For this review, take the finished solid that the model builds, in its own axes (mm). A direction names the side the tool comes from. Coordinates: 2 decimals unless noted, no trailing zeros. Write each loop counter-clockwise with the first axis right and the second up, starting at its lowest first coordinate (ties: lowest second). Pieces come first, ordered by that corner, then holes.
```python
from build123d import *

# Parameters (mm, degrees)
SKETCH_1_W          = 50
SKETCH_1_H          = 29.5
SKETCH_1_R          = 1.75
EXTRUDE_1_DEPTH     = 5
SKETCH_1_17_R       = 3.1
CUT_EXTRUDE_1_DEPTH = 2.6
EXTRUDE_START       = 5
SKETCH_1_18_W       = 50
SKETCH_1_18_H       = 4
SKETCH_1_18_W_2     = 15
EXTRUDE_2_DEPTH     = 49
SKETCH_2_R          = 1.5
CUT_EXTRUDE_2_DEPTH = 76.968743573
SKETCH_2_4_R        = 2.25
CUT_EXTRUDE_3_DEPTH = 2
SKETCH_4_R          = 1.5
CUT_EXTRUDE_4_DEPTH = 75.553671942
SKETCH_4_3_R        = 2.25
CUT_EXTRUDE_5_DEPTH = 2
SKETCH_5_W          = 35
SKETCH_5_H          = 4
EXTRUDE_4_DEPTH     = 32
SKETCH_6_R          = 1.5
CUT_EXTRUDE_6_DEPTH = 97.944571792
SKETCH_6_3_R        = 2.25
CUT_EXTRUDE_7_DEPTH = 2


with BuildPart() as part:
    # 草图1 → 凸台-拉伸1 (new body)
    with BuildSketch(Plane(origin=(0, 0, 0), x_dir=(1, 0, 0), z_dir=(0, 1, 0))):
        with Locations((25, -14.75)):
            Rectangle(SKETCH_1_W, SKETCH_1_H)
        with Locations(Location((23.4, -12, 0), (0, 0, 270))):
            Circle(SKETCH_1_R, mode=Mode.SUBTRACT)
        with Locations(Location((44.400952359, -19.4, 0), (0, 0, 270))):
            Circle(SKETCH_1_R, mode=Mode.SUBTRACT)
    extrude(amount=EXTRUDE_1_DEPTH)

    # 草图1<17> → 切除-拉伸1 (cut)
    with BuildSketch(Plane(origin=(0, 0, 0), x_dir=(1, 0, 0), z_dir=(0, 1, 0))):
        with Locations(Location((23.4, -12, 0), (0, 0, 270))):
            Circle(SKETCH_1_17_R)
        with Locations(Location((44.400952359, -19.4, 0), (0, 0, 270))):
            Circle(SKETCH_1_17_R)
    extrude(amount=CUT_EXTRUDE_1_DEPTH, mode=Mode.SUBTRACT)

    # 草图1<18> → 凸台-拉伸2 (add)
    with BuildSketch(Plane(origin=(0, 0, 0), x_dir=(1, 0, 0), z_dir=(0, 1, 0)).offset(EXTRUDE_START)):
        with Locations((25, 2)):
            Rectangle(SKETCH_1_18_W, SKETCH_1_18_H)
        with Locations((7.5, 2)):
            Rectangle(SKETCH_1_18_W_2, SKETCH_1_18_H)
    extrude(amount=-EXTRUDE_2_DEPTH)

    # 草图2 → 切除-拉伸2 (cut, through all)
    with BuildSketch(Plane(origin=(0, 5, 0), x_dir=(1, 0, 0), z_dir=(0, 1, 0))):
        with Locations(Location((5, -24.5, 0), (0, 0, 270))):
            Circle(SKETCH_2_R)
        with Locations(Location((5, -6, 0), (0, 0, 270))):
            Circle(SKETCH_2_R)
    extrude(amount=-CUT_EXTRUDE_2_DEPTH, mode=Mode.SUBTRACT)

    # 草图2<4> → 切除-拉伸3 (cut)
    with BuildSketch(Plane(origin=(0, 5, 0), x_dir=(1, 0, 0), z_dir=(0, 1, 0))):
        with Locations(Location((5, -24.5, 0), (0, 0, 270))):
            Circle(SKETCH_2_4_R)
        with Locations(Location((5, -6, 0), (0, 0, 270))):
            Circle(SKETCH_2_4_R)
    extrude(amount=-CUT_EXTRUDE_3_DEPTH, mode=Mode.SUBTRACT)

    # 草图4 → 切除-拉伸4 (cut, through all)
    with BuildSketch(Plane(origin=(0, 0, -4), x_dir=(-1, 0, 0), z_dir=(0, 0, -1))):
        with Locations((-5, -29)):
            Circle(SKETCH_4_R)
    extrude(amount=-CUT_EXTRUDE_4_DEPTH, mode=Mode.SUBTRACT)

    # 草图4<3> → 切除-拉伸5 (cut)
    with BuildSketch(Plane(origin=(0, 0, -4), x_dir=(-1, 0, 0), z_dir=(0, 0, -1))):
        with Locations((-5, -29)):
            Circle(SKETCH_4_3_R)
    extrude(amount=-CUT_EXTRUDE_5_DEPTH, mode=Mode.SUBTRACT)

    # 草图5 → 凸台-拉伸4 (add)
    with BuildSketch(Plane.XZ.offset(44)):
        with Locations((32.5, -2)):
            Rectangle(SKETCH_5_W, SKETCH_5_H)
    extrude(amount=EXTRUDE_4_DEPTH)

    # 草图6 → 切除-拉伸6 (cut, through all)
    with BuildSketch(Plane(origin=(0, 0, -4), x_dir=(-1, 0, 0), z_dir=(0, 0, -1))):
        with Locations((-22, -69)):
            Circle(SKETCH_6_R)
        with Locations((-43, -51)):
            Circle(SKETCH_6_R)
    extrude(amount=-CUT_EXTRUDE_6_DEPTH, mode=Mode.SUBTRACT)

    # 草图6<3> → 切除-拉伸7 (cut)
    with BuildSketch(Plane(origin=(0, 0, -4), x_dir=(-1, 0, 0), z_dir=(0, 0, -1))):
        with Locations((-22, -69)):
            Circle(SKETCH_6_3_R)
        with Locations((-43, -51)):
            Circle(SKETCH_6_3_R)
    extrude(amount=-CUT_EXTRUDE_7_DEPTH, mode=Mode.SUBTRACT)


solid = part.part
```
Q1. For probe 1 along Z at (x, y) = (23.4, 4.4); probe 2 along Y at (x, z) = (43, -0.6); probe 3 along X at (y, z) = (3.5, 24.5), list the stretches that pass through material, from the lowest coordinate up.
Ans:
probe 1: z = -4 to 10.25, 13.75 to 29.5
probe 2: y = -76 to -52.5, -49.5 to 5
probe 3: x = 0 to 2.75, 7.25 to 50
Q2. Add section D-D (z = 2). State the section outline as (x, y) points, then the cut area to 3 significant figures.
Ans:
outline: (0, 0) - (50, 0) - (50, 5) - (0, 5) - close
area: 250 mm2
Q3. Add section A-A (y = -29). State the section outline as (x, z) points.
Ans:
outline: (0, -4) - (2.75, -4) - (2.75, -2) - (3.5, -2) - (3.5, 0) - (0, 0) - close; (6.5, -2) - (7.25, -2) - (7.25, -4) - (50, -4) - (50, 0) - (6.5, 0) - close
Q4. Add section C-C (x = 17.5). State the section outline as (y, z) points.
Ans:
outline: (-76, -4) - (5, -4) - (5, 29.5) - (0, 29.5) - (0, 0) - (-76, 0) - close
Q5. Clearance check with flat-ended pins moving along their axes: pin 1 Ø6 at (x, z) = (5, 24.5) entering from +Y; pin 2 Ø4.5 at (x, z) = (23.4, 12) entering from -Y; pin 3 Ø4 at (x, z) = (5, 6) entering from +Y; pin 4 Ø6 at (x, y) = (43, -51) entering from +Z. State where each tip first meets the part, or that it passes through.
Ans:
pin 1: stops at y = 5
pin 2: stops at y = 2.6
pin 3: stops at y = 3
pin 4: stops at z = 0
Q6. Add section B-B (z = 24.5). State the section outline as (x, y) points.
Ans:
outline: (0, 0) - (3.5, 0) - (3.5, 3) - (2.75, 3) - (2.75, 5) - (0, 5) - close; (6.5, 0) - (50, 0) - (50, 5) - (7.25, 5) - (7.25, 3) - (6.5, 3) - close
Q7. Tool access review of faces 4 (the flat face through (7, -44, -2)), 5 (the cylindrical face through (25.5, 1.28, 9.72)), 6 (the cylindrical face through (43.29, -48.77, -3.01)), 7 (the cylindrical face through (44.48, 3.78, 17.65)), 8 (the flat face through (25, 0, 18)): name each direction out of +Z, -Z, +X, -X, +Y, -Y from which nothing blocks a thin tool from reaching the whole face with its end or side.
Ans:
face 4: +Z, -Z, -X, -Y
face 5: -Y
face 6: -Z
face 7: +Y, -Y
face 8: +Z, +X, -X, -Y
Q8. Draft analysis for pull direction Y (two halves, no side actions). For faces 1 (the flat face through (43, -49, -2)), 2 (the flat face through (30, -37, 0)), 3 (the flat face through (7, 3, 6)), state which applies: +Y half, -Y half, draft (parallel to the pull), parting line (faces both ways), or undercut.
Ans:
face 1: undercut
face 2: draft
face 3: +Y half
